The listing builds one solid part. Answer for the finished solid, in the listing's coordinates (mm). Face numbers are marked on the shaded views. Round coordinates to 2 decimals unless told otherwise and drop trailing zeros. Write each loop counter-clockwise with the first axis right and the second up, starting at its lowest first coordinate (ties: lowest second). Pieces come first, ordered by that corner, then holes.
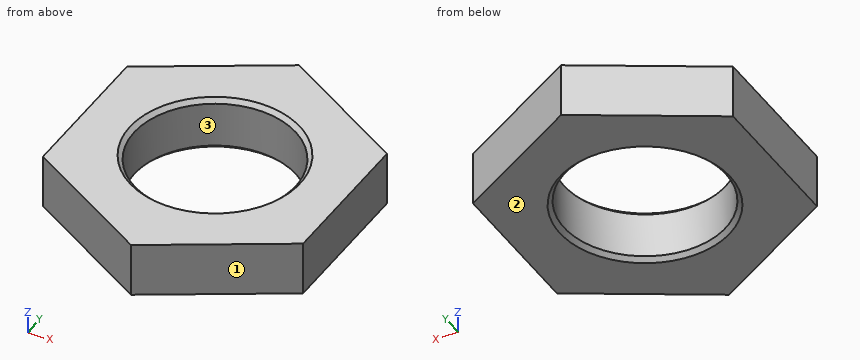
from build123d import *

# Parameters (mm, degrees)
EXTRUDE_1_DEPTH     = 2.5
SKETCH_3_R          = 3.724956963
CUT_EXTRUDE_1_DEPTH = 6.5
CHAMFER_1_SIZE      = 0.2


with BuildPart() as part:
    # 草图2 → 凸台-拉伸1 (new body)
    with BuildSketch(Plane.XY):
        Polygon((0, 6.92820323), (-6, 3.464101615), (-6, -3.464101615), (0, -6.92820323), (6, -3.464101615), (6, 3.464101615), align=None)
    extrude(amount=EXTRUDE_1_DEPTH)

    # 草图3 → 切除-拉伸1 (cut)
    with BuildSketch(Plane(origin=(0, 0, 0), x_dir=(-1, 0, 0), z_dir=(0, 0, -1))):
        Circle(SKETCH_3_R)
    extrude(amount=-CUT_EXTRUDE_1_DEPTH, mode=Mode.SUBTRACT)

    # 倒角1
    chamfer_1_edges = [part.edges().sort_by_distance(p)[0] for p in [
        (3.724956963, 0, 2.5),
        (3.724956963, 0, 0),
    ]]
    chamfer(chamfer_1_edges, length=CHAMFER_1_SIZE)


solid = part.part
1. For a pull along Y with two mould halves and no side action, classify the marked faces 1, 2 and 3 as released by +Y, released by -Y, zero draft, split by the parting line, or undercut.
Geometry says:
face 1: released by -Y
face 2: zero draft
face 3: undercut
2. Straight lines are drawn through the part: line 1 along X through (y, z) = (-1, 0.65); line 2 along Y through (x, z) = (-0.75, 2.45); line 3 along X through (y, z) = (-3.25, 1.1). For each, find the intervals that lie inside material, in ascending order.
Geometry says:
line 1: x = -6 to -3.59, 3.59 to 6
line 2: y = -6.5 to -3.8, 3.8 to 6.5
line 3: x = -6 to -1.82, 1.82 to 6
3. Section B-B on z = 2.05 is taken. Determine the outline of the cut face in (x, y), plus the area to 3 significant figures.
Geometry says:
outline: (-6, -3.46) - (0, -6.93) - (6, -3.46) - (6, 3.46) - (0, 6.93) - (-6, 3.46) - close; hole circle Ø7.45 at (0, 0)
area: 81.1 mm2
4. Section A-A on y = 0 is taken. Determine the outline of the cut face in (x, z).
Geometry says:
outline: (-6, 0) - (-3.92, 0) - (-3.72, 0.2) - (-3.72, 2.3) - (-3.92, 2.5) - (-6, 2.5) - close; (3.72, 0.2) - (3.92, 0) - (6, 0) - (6, 2.5) - (3.92, 2.5) - (3.72, 2.3) - close
5. Given pin 1 (1 mm diameter, centred on x = -3, z = 1, fed in from -Y), flat-ended and moving along its own axis, determine where the tip first touches the part or whether it passes through.
Geometry says:
pin 1: stops at y = -5.48
6. Section C-C on y = -5.25 is taken. Determine the outline of the cut face in (x, z), plus the area to 3 significant figures.
Geometry says:
outline: (-2.91, 0) - (2.91, 0) - (2.91, 2.5) - (-2.91, 2.5) - close
area: 14.5 mm2
7. Section D-D on y = 4.25 is taken. Determine the outline of the cut face in (x, z), plus the area to 3 significant figures.
Geometry says:
outline: (-4.64, 0) - (4.64, 0) - (4.64, 2.5) - (-4.64, 2.5) - close
area: 23.2 mm2
